Geometry check sheet. Reference: drawing and pictorial views, mm from the part's lowest x, y, z. A direction names the side the tool comes from. Round coordinates to 2 decimals unless told otherwise and drop trailing zeros. Order: outer loops, then holes, each group sorted by start corner. A loop starts at its lowest first (then second) coordinate and runs counter-clockwise, first axis right, second up.
(1) Material ranges on line 1 along Z through (x, y) = (27.5, 3.05); line 2 along X through (y, z) = (4.45, 13); line 3 along X through (y, z) = (3.2, 13.75), recorded low to high.
(2) Go/stop test with flat-tipped pins: pin 1 (4 mm diameter, centred on x = 5, z = 12.73, fed in from +Y); pin 2 (8 mm diameter, centred on x = 20.5, z = 21.5, fed in from -Y). Record where each tip stops, or that it passes through.
(3) Sectioned sample at D-D (z = 18.75). Record the boundary of the cut face in (x, y).
(4) Sectioned sample at A-A (x = 27.5). Record the boundary of the cut face in (y, z).
(5) Sectioned sample at C-C (x = 50). Record the boundary of the cut face in (y, z).
(6) Sectioned sample at B-B (y = 1.95). Record the boundary of the cut face in (x, z).
(7) Set-up check for the marked faces 1 and 2: record each of +Z, -Z, +X, -X, +Y, -Y from which the full face is reachable in a straight line by a thin tool's end or side.
(8) Release check for a two-part mould opening along Z. For the marked faces 3, 4 and 5 record: +Z half, -Z half, draft (parallel to the pull), parting line (faces both ways), or undercut.
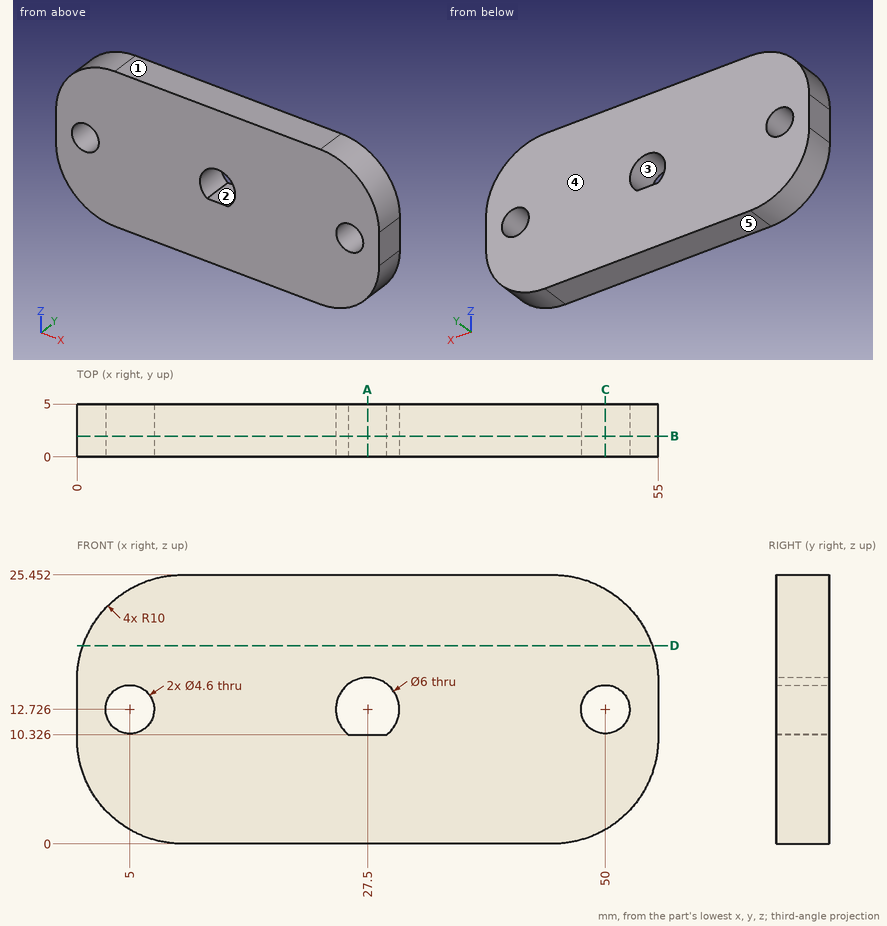
Answer below:
1. line 1: z = 0 to 10.33, 15.73 to 25.45
1. line 2: x = 0 to 2.72, 7.28 to 24.51, 30.49 to 47.72, 52.28 to 55
1. line 3: x = 0 to 2.94, 7.06 to 24.68, 30.32 to 47.94, 52.06 to 55
2. pin 1: passes through
2. pin 2: stops at y = 0
3. outline: (0.56, 0) - (54.44, 0) - (54.44, 5) - (0.56, 5) - close
4. outline: (0, 0) - (5, 0) - (5, 10.33) - (0, 10.33) - close; (0, 15.73) - (5, 15.73) - (5, 25.45) - (0, 25.45) - close
5. outline: (0, 1.34) - (5, 1.34) - (5, 10.43) - (0, 10.43) - close; (0, 15.03) - (5, 15.03) - (5, 24.11) - (0, 24.11) - close
6. outline: (0, 10) arc R10 ccw to (10, 0) - (45, 0) arc R10 ccw to (55, 10) - (55, 15.45) arc R10 ccw to (45, 25.45) - (10, 25.45) arc R10 ccw to (0, 15.45) - close; hole circle Ø4.6 at (5, 12.73); hole (25.7, 10.33) - (29.3, 10.33) arc R3 ccw (long way) to start; hole circle Ø4.6 at (50, 12.73)
7. face 1: +Z, +X, -X, +Y, -Y
7. face 2: +Y, -Y
8. face 3: undercut
8. face 4: draft
8. face 5: -Z half
